CAD build for the part. Positions are in the model's coordinates, mm. A direction names the side the tool comes from. Give positions to 0.01 mm unless a question says otherwise; leave off trailing zeros. Write each loop counter-clockwise with the first axis right and the second up, starting at its lowest first coordinate (ties: lowest second). Pieces come first, ordered by that corner, then holes. Notation, with made-up numbers: (83.25, 32.5) -> (120.25, 32.5) arc R10 cw to (120.25, 41.5) -> close; hole circle Ø6 at (73, 2.5). An arc over 180 degrees is marked (long way). Answer in a Markdown table with one row per item. Add a question column.
Autodesk Inventor part; units mm, degrees
ref_plane "YZ Plane" through (0, 0, 0) normal (1, 0, 0) x (0, 1, 0)
ref_plane "XZ Plane" through (0, 0, 0) normal (0, 1, 0) x (-1, 0, 0)
ref_plane "XY Plane" through (0, 0, 0) normal (0, 0, 1) x (1, 0, 0)
sketch "Sketch1" plane through (0, 0, 0) normal (0, 0, 1) x (1, 0, 0)
  line L0 (-75, 45) -> (75, 45)
  line L1 (75, 45) -> (75, -45)
  line L2 (75, -45) -> (-75, -45)
  line L3 (-75, -45) -> (-75, 45)
  line L4 (-75, 45) -> (75, -45) construction
  line L5 (75, 45) -> (-75, -45) construction
  point P0 (0, 0)
  dimension "d0" = 150
  dimension "d1" = 90
extrude "Extrusion1" add sketch "Sketch1" along normal blind 5
fillet "Fillet1" radius 5 4 edges at (75, 45, 2.5) (75, -45, 2.5) (-75, -45, 2.5) (-75, 45, 2.5)
sketch "Sketch2" plane through (0, 0, 5) normal (0, 0, 1) x (1, 0, 0)
  line L0 (-61.6, -36.6) -> (61.6, -36.6)
  line L1 (66.6, -31.6) -> (66.6, 31.6)
  line L2 (61.6, 36.6) -> (-61.6, 36.6)
  line L3 (-66.6, 31.6) -> (-66.6, -31.6)
  line L4 (-66.6, -36.6) -> (66.6, 36.6) construction
  line L5 (66.6, -36.6) -> (-66.6, 36.6) construction
  arc A0 (-61.6, 36.6) -> (-66.6, 31.6) centre (-61.6, 31.6) ccw
  arc A1 (-66.6, -31.6) -> (-61.6, -36.6) centre (-61.6, -31.6) ccw
  arc A2 (61.6, -36.6) -> (66.6, -31.6) centre (61.6, -31.6) ccw
  arc A3 (66.6, 31.6) -> (61.6, 36.6) centre (61.6, 31.6) ccw
  point P0 (0, 0)
  dimension "d5" = 133.2
  dimension "d6" = 73.2
  dimension "d9" = 5
extrude "Extrusion2" cut sketch "Sketch2" against normal blind 5
sketch "Sketch3" plane through (0, 0, 5) normal (0, 0, 1) x (1, 0, 0)
  line L0 (66.6, 31.6) -> (66.6, -31.6)
  line L1 (66.6, 0) -> (75, 0) construction
  line L2 (75, -40) -> (75, 40)
  line L3 (70.8, 0) -> (70.8, 28.8336) construction
  circle A0 centre (70.8, 28.8336) radius 3.25
  point P0 (0, 0)
  dimension "d10" = 6.5
extrude "Extrusion3" cut sketch "Sketch3" against normal blind 2.4
sketch "Sketch4" plane through (70.8, 28.8336, 2.6) normal (0, 0, 1) x (1, 0, 0)
  circle A0 centre (0, 0) radius 2
  point P0 (-70.8, -28.8336)
  dimension "d13" = 4
extrude "Extrusion4" cut sketch "Sketch4" against normal blind 15
sketch "Sketch7" plane through (0, 0, 3) normal (0, 0, 1) x (1, 0, 0)
  line L0 (-66.6, -31.6) -> (-66.6, 31.6)
  line L1 (-66.6, 0.4) -> (-51.6, 0.4) construction
  line L2 (61.6, -36.6) -> (-61.6, -36.6)
  line L3 (-51.6, -36.6) -> (-51.6, -19.6) construction
  line L4 (-51.6, -36.6) -> (-34.6, -36.6) construction
  line L5 (-66.6, 19.9067) -> (-31.6, 19.9067) construction
  line L6 (-31.6, -17.6) -> (-31.6, 19.4) construction
  line L7 (-31.6, -36.6) -> (5.4, -36.6) construction
  line L8 (-49.6, -19.6) -> (-33.6, -19.6)
  line L9 (-31.6, -19.6) -> (-31.6, 17.4)
  line L10 (-33.6, 19.4) -> (-49.6, 19.4)
  line L11 (-51.6, 17.4) -> (-51.6, -17.6)
  arc A0 (-49.6, 19.4) -> (-51.6, 17.4) centre (-49.6, 17.4) ccw
  arc A1 (-31.6, 17.4) -> (-33.6, 19.4) centre (-33.6, 17.4) ccw
  arc A2 (-33.6, -19.6) -> (-31.6, -17.6) centre (-33.6, -17.6) ccw
  arc A3 (-51.6, -17.6) -> (-49.6, -19.6) centre (-49.6, -17.6) ccw
  point P0 (0, 0)
  point P1 (-67, -23.834)
  point P2 (-31.6, -17.6)
  dimension "d30" = 17
  dimension "d31" = 90
  dimension "d34" = 56
  dimension "d35" = 90
  dimension "d36" = 15
  dimension "d37" = 35
  dimension "d38" = 2
extrude "Extrusion6" [suppressed]
properties part number "Frame"
Item 1: Probe L1, parallel to X at y = 28.5, z = 2.15; L2, parallel to X at y = -21, z = 2.55; L3, parallel to Y at x = -6.5, z = 0.4. List the from-to ranges inside material, lowest first. Write a range as from..to.
Item 2: Slice it at B-B, the plane x = -35. List the corners of the cut face in (y, z), then the cut area to 3 significant figures.
Item 3: Mould opens along X. For faces 4 (the face through (-66.6, 0, 3)), 5 (the face through (-6, 37, 0)), 6 (the face through (71.875, 30.52, 1.318)), 7 (the face through (75, 1, 2)) say: released by +X, released by -X, zero draft, split by the parting line, or undercut.
Item 4: Drop flat-ended pins along their axis: pin 1 Ø4.5 at (x, y) = (70.8, 28.83) entering from -Z; pin 2 Ø6 at (x, y) = (70.8, 28.83) entering from +Z. Give the stop position or say it passes through.
Item 5: Slice it at A-A, the plane y = -21.5. List the corners of the cut face in (x, z), then the cut area to 3 significant figures.
Item 6: Which spindle directions (+Z, -Z, +X, -X, +Y, -Y) get a long thin tool onto all of the face, cutting with end or side? Do faces 1 (the face through (65.17, 35.1, 2.54)), 2 (the face through (73.9, 29.81, 3.82)), 3 (the face through (74, 43, 3)). Say none if no direction does.
Item 7: Slice it at C-C, the plane z = 3.4. List the corners of the cut face in (x, y).
Answer key:
| question | item | result |
|---|---|---|
| 1 | L1 | x = -75..-66.6, 66.6..68.83, 72.77..75 |
| 1 | L2 | x = -75..-66.6, 66.6..75 |
| 1 | L3 | y = -45..-36.6, 36.6..45 |
| 2 | outline | (-45, 0) -> (-36.6, 0) -> (-36.6, 5) -> (-45, 5) -> close; (36.6, 0) -> (45, 0) -> (45, 5) -> (36.6, 5) -> close |
| 2 | area | 84.0 mm² |
| 3 | face 4 | undercut |
| 3 | face 5 | zero draft |
| 3 | face 6 | undercut |
| 3 | face 7 | released by +X |
| 4 | pin 1 | stops at z = 0 |
| 4 | pin 2 | stops at z = 2.6 |
| 5 | outline | (-75, 0) -> (-66.6, 0) -> (-66.6, 5) -> (-75, 5) -> close; (66.6, 0) -> (75, 0) -> (75, 5) -> (66.6, 5) -> close |
| 5 | area | 84.0 mm² |
| 6 | face 1 | +Z, -Z |
| 6 | face 2 | +Z |
| 6 | face 3 | +Z, -Z, +X, +Y |
| 7 | outline | (-75, -40) arc R5 ccw to (-70, -45) -> (70, -45) arc R5 ccw to (75, -40) -> (75, 40) arc R5 ccw to (70, 45) -> (-70, 45) arc R5 ccw to (-75, 40) -> close; hole (-66.6, -31.6) arc R5 ccw to (-61.6, -36.6) -> (61.6, -36.6) arc R5 ccw to (66.6, -31.6) -> (66.6, 31.6) arc R5 ccw to (61.6, 36.6) -> (-61.6, 36.6) arc R5 ccw to (-66.6, 31.6) -> close; hole circle Ø6.5 at (70.8, 28.83) |
